Part model, mm, in its own coordinate system. Give positions to 0.01 mm unless a question says otherwise; leave off trailing zeros. Order: outer loops, then holes, each group sorted by start corner. A loop starts at its lowest first (then second) coordinate and runs counter-clockwise, first axis right, second up. Notation, with made-up numbers: M 1,-22.75 L 45,-22.75 A19 ccw 45,10.25 Z; hole C 36,47.25 d6. An arc over 180 degrees is marked long. Answer as a JSON object with one key per item and string values.
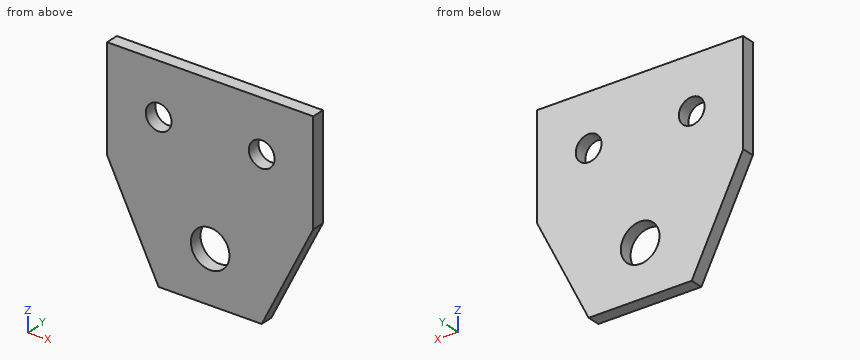
Autodesk Inventor part; units mm, degrees
ref_plane "YZ Plane" through (0, 0, 0) normal (1, 0, 0) x (0, 1, 0)
ref_plane "XZ Plane" through (0, 0, 0) normal (0, 1, 0) x (-1, 0, 0)
ref_plane "XY Plane" through (0, 0, 0) normal (0, 0, 1) x (1, 0, 0)
sketch "Sketch1" plane through (0, 0, 0) normal (0, 1, 0) x (-1, 0, 0)
  line L0 (0, 0) -> (50.8, 0)
  line L1 (50.8, 0) -> (50.8, -25.4)
  line L2 (50.8, -25.4) -> (38.1, -50.8)
  line L3 (38.1, -50.8) -> (12.7, -50.8)
  line L4 (12.7, -50.8) -> (0, -25.4)
  line L5 (0, -25.4) -> (0, 0)
  circle A0 centre (12.7, -12.7) radius 3.175
  circle A1 centre (38.1, -12.7) radius 3.175
  circle A2 centre (25.4, -38.1) radius 4.7625
  dimension "d0" = 25.4
  dimension "d1" = 50.8
  dimension "d2" = 25.4
  dimension "d3" = 50.8
  dimension "d4" = 12.7
  dimension "d5" = 6.35
  dimension "d6" = 6.35
  dimension "d7" = 12.7
  dimension "d8" = 12.7
  dimension "d9" = 12.7
  dimension "d10" = 12.7
  dimension "d11" = 9.525
  dimension "d12" = 12.7
  dimension "d13" = 12.7
extrude "Extrusion1" add sketch "Sketch1" along normal blind 3.175
properties part number "15102898-16-P-0212"
1. Pin check, flat tips, straight feed: P1, Ø4, axis at x = -38.1, z = -12.7, coming from the -Y side; P2, Ø1.5, axis at y = 1.5, z = -37, coming from the -X side (3 decimals). Stop position of each tip, or through.
Worked answers:
{"P1": "passes through", "P2": "stops at x = -45.375"}
2. Cut at D-D on z = -35.5. Give the cut face in (x, y) (3 decimals), plus the area to 3 significant figures.
Worked answers:
{"outline": "M -45.75,0 L -29.39,0 L -29.39,3.175 L -45.75,3.175 Z; M -21.41,0 L -5.05,0 L -5.05,3.175 L -21.41,3.175 Z", "area": "104 mm^2"}
3. Probe line 1 along Z through (x, y) = (-13, 2.7); line 2 along X through (y, z) = (1.5, -14); line 3 along Z through (x, y) = (-25.4, 1.6). List the from-to ranges inside material, lowest first.
Worked answers:
{"line 1": "z = -50.8 to -15.86, -9.54 to 0", "line 2": "x = -50.8 to -41, -35.2 to -15.6, -9.8 to 0", "line 3": "z = -50.8 to -42.86, -33.34 to 0"}
4. Cut at B-B on x = -25.4. Give the cut face in (y, z) (1 decimal), plus the area to 3 significant figures.
Worked answers:
{"outline": "M 0,-50.8 L 3.2,-50.8 L 3.2,-42.9 L 0,-42.9 Z; M 0,-33.3 L 3.2,-33.3 L 3.2,0 L 0,0 Z", "area": "131 mm^2"}
5. Cut at A-A on z = -12.7. Give the cut face in (x, y) (3 decimals), plus the area to 3 significant figures.
Worked answers:
{"outline": "M -50.8,0 L -41.275,0 L -41.275,3.175 L -50.8,3.175 Z; M -34.925,0 L -15.875,0 L -15.875,3.175 L -34.925,3.175 Z; M -9.525,0 L 0,0 L 0,3.175 L -9.525,3.175 Z", "area": "121 mm^2"}
6. Cut at C-C on y = 2.25. State how many separate pieces and enclosed holes the cut face has, plus the area to 3 significant figures.
Worked answers:
{"separate pieces": "1", "enclosed holes": "3", "area": "2,120 mm^2"}
